Drawing for the job (mm, zero at the part's lowest x, y, z). A direction names the side the tool comes from. Give positions to 0.01 mm unless a question says otherwise; leave off trailing zeros. Order: outer loops, then holes, each group sorted by start corner. A loop starts at its lowest first (then second) coordinate and runs counter-clockwise, first axis right, second up. Notation, with made-up numbers: (-39.5, -9) -> (-19.5, -9) arc R25 cw to (-19.5, 13) -> close; hole circle Ø6 at (43, 26). An arc over 180 degrees is marked (long way). One line per item, written item: value. Start each with the question number.
(1) Saw through at B-B on z = 14. Give the cut face in (x, y) (3 decimals), plus the area to 3 significant figures.
(2) Which spindle directions (+Z, -Z, +X, -X, +Y, -Y) get a long thin tool onto all of the face, cutting with end or side? Do the marked faces 4 and 5. Say none if no direction does.
(3) Saw through at A-A on x = 14.5. Give the cut face in (y, z).
(4) Probe line 1 (Z direction, x = 3.25, y = 18.25); line 2 (Z direction, x = 4.25, y = 9.5); line 3 (Z direction, x = 12.75, y = 17) (1 decimal). List the from-to ranges inside material, lowest first.
(5) Saw through at C-C on y = 8. Give the cut face in (x, z), plus the area to 3 significant figures.
(6) Two-plate mould, pull along Z, no slides. Class the marked faces 1, 2 and 3: +Z half, -Z half, draft (parallel to the pull), parting line (faces both ways), or undercut.
(7) Pin check, flat tips, straight feed: pin 1 (3 mm diameter, centred on x = 7, y = 8, fed in from +Z); pin 2 (12 mm diameter, centred on y = 8.5, z = 3.5, fed in from +X); pin 3 (8 mm diameter, centred on x = 7.5, y = 5, fed in from +Z); pin 4 (5 mm diameter, centred on x = 11, z = 6, fed in from -Y). Stop position of each tip, or through.
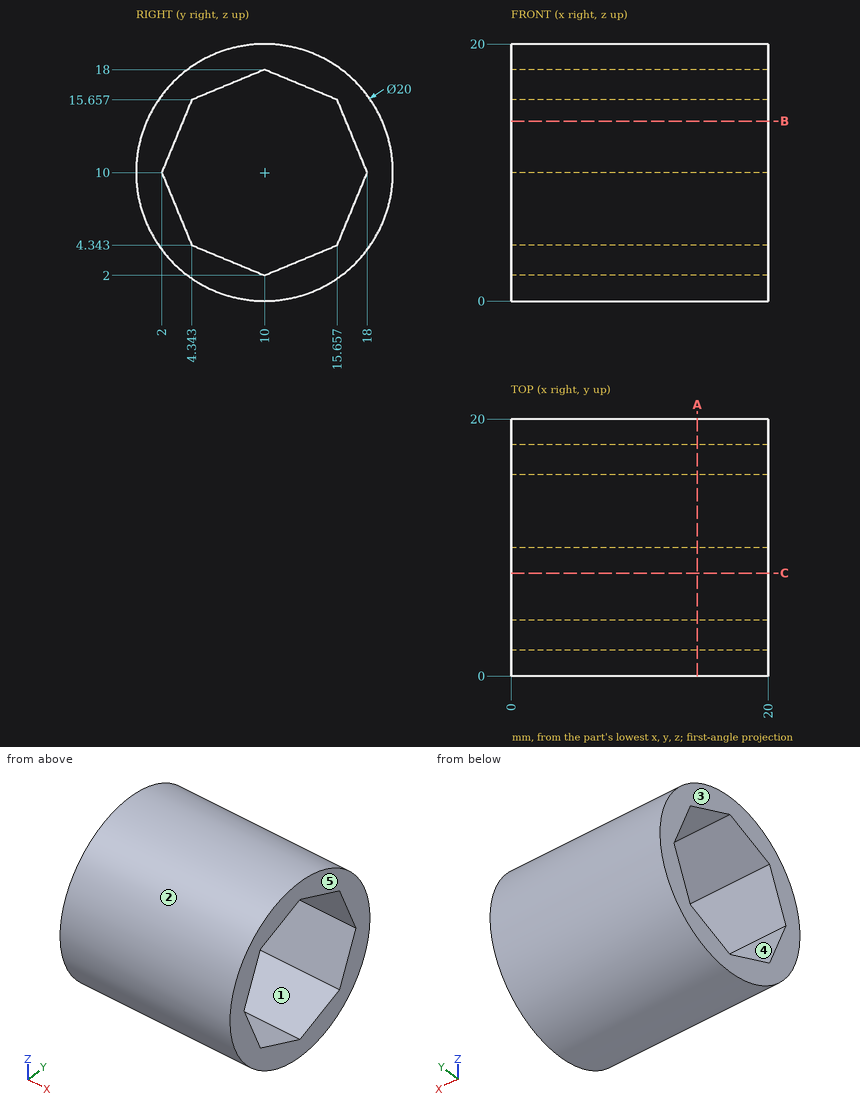
Results below:
1. outline: (0, 0.835) -> (20, 0.835) -> (20, 3.657) -> (0, 3.657) -> close; (0, 16.343) -> (20, 16.343) -> (20, 19.165) -> (0, 19.165) -> close
1. area: 113 mm²
2. face 4: +X, -X
2. face 5: +Z, -Z, +X, +Y, -Y
3. outline: circle Ø20 at (10, 10); hole (2, 10) -> (4.34, 4.34) -> (10, 2) -> (15.66, 4.34) -> (18, 10) -> (15.66, 15.66) -> (10, 18) -> (4.34, 15.66) -> close
4. line 1: z = 4.35 to 15.65
4. line 2: z = 0.01 to 2.21, 17.79 to 19.99
4. line 3: z = 2.9 to 7.6, 12.4 to 17.1
5. outline: (0, 0.2) -> (20, 0.2) -> (20, 2.83) -> (0, 2.83) -> close; (0, 17.17) -> (20, 17.17) -> (20, 19.8) -> (0, 19.8) -> close
5. area: 105 mm²
6. face 1: undercut
6. face 2: parting line
6. face 3: draft
7. pin 1: stops at z = 19.99
7. pin 2: stops at x = 20
7. pin 3: stops at z = 19.95
7. pin 4: stops at y = 0.11
